Geometry check sheet. Reference: the model listing, model coordinates, mm. A direction names the side the tool comes from. Give positions to 0.01 mm unless a question says otherwise; leave off trailing zeros. Loops run counter-clockwise (first coordinate to the right, second up) from the corner with the lowest first, then second, coordinate; pieces in that order, holes last. Notation, with made-up numbers: (29.25, 69.5) -> (65.25, 69.5) arc R27 cw to (65.25, 90.5) -> close; hole circle Ø4 at (-24, 15.25). An arc over 180 degrees is marked (long way). One line per item, written item: value. Start each with the question number.
(1) Draft check along Z on faces 4 (the face through (0, 5, -33)), 5 (the face through (-4, 11.5, -18)), 6 (the face through (0, 7, -2)). Enter one of: pulls with the +Z half, pulls with the -Z half, needs draft (parallel to the pull), parting line crosses it, or undercut.
(2) Sectioned sample at D-D, the plane x = 0.25. Record the cut outline in (y, z), then the cut area to 3 significant figures.
(3) Gauge pin test, flat ends, axial feed: pin 1 Ø4.5 at (x, z) = (1, 0) entering from +Y; pin 2 Ø1.2 at (y, z) = (13, 0.5) entering from -X. Record the tip position at first contact, or that the pin passes through.
(4) Tool access check on faces 1 (the face through (0, 7, 2)), 2 (the face through (3.5, 13, 0)), 3 (the face through (-10.5, 2, 0)). Record the directions out of +Z, -Z, +X, -X, +Y, -Y that give a thin tool (end or side, any length) a straight path to the whole face; none if there is none.
(5) Sectioned sample at A-A, the plane y = 7.5. Record the cut outline in (x, z), then the cut area to 3 significant figures.
(6) Scan lines: line 1 along Z through (x, y) = (-1, 9); line 2 along X through (y, z) = (12.75, 9.5); line 3 along Y through (x, z) = (0, -21). Record each from-to range of solid material in increasing order. Write a range as from..to.
(7) Sectioned sample at C-C, the plane z = -0.5. Record the cut outline in (x, y), then the cut area to 3 significant figures.
(8) Sectioned sample at B-B, the plane x = 5.75. Record the cut outline in (y, z), then the cut area to 3 significant figures.
from build123d import *

# Parameters (mm, degrees)
SK_P01_CARRIER_W             = 21
SK_P01_CARRIER_H             = 66
P01_CARRIER_DEPTH            = 3
P02_WAGO221415GNDSTAR_START  = 3
SK_P02_WAGO221415GNDSTAR_W   = 21
SK_P02_WAGO221415GNDSTAR_H   = 31
P02_WAGO221415GNDSTAR_DEPTH  = 8.5
P03_WAGO221415PACKNODE_START = 3
SK_P03_WAGO221415PACKNODE_W  = 21
SK_P03_WAGO221415PACKNODE_H  = 31
P03_WAGO221415PACKNODE_DEPTH = 8.5
P04_LEVERS_START             = 11.5
SK_P04_LEVERS_W              = 7
SK_P04_LEVERS_H              = 66
P04_LEVERS_DEPTH             = 2.5


with BuildPart() as part:
    # SK_P01_Carrier → P01_Carrier (new body)
    with BuildSketch(Plane(origin=(0, 0, 0), x_dir=(1, 0, 0), z_dir=(0, 1, 0))):
        Rectangle(SK_P01_CARRIER_W, SK_P01_CARRIER_H)
    extrude(amount=P01_CARRIER_DEPTH)

    # SK_P02_WAGO221415GNDstar → P02_WAGO221415GNDstar (add)
    with BuildSketch(Plane(origin=(0, 0, 0), x_dir=(1, 0, 0), z_dir=(0, 1, 0)).offset(P02_WAGO221415GNDSTAR_START)):
        with Locations((0, 17.5)):
            Rectangle(SK_P02_WAGO221415GNDSTAR_W, SK_P02_WAGO221415GNDSTAR_H)
    extrude(amount=P02_WAGO221415GNDSTAR_DEPTH)

    # SK_P03_WAGO221415packnode → P03_WAGO221415packnode (add)
    with BuildSketch(Plane(origin=(0, 0, 0), x_dir=(1, 0, 0), z_dir=(0, 1, 0)).offset(P03_WAGO221415PACKNODE_START)):
        with Locations((0, -17.5)):
            Rectangle(SK_P03_WAGO221415PACKNODE_W, SK_P03_WAGO221415PACKNODE_H)
    extrude(amount=P03_WAGO221415PACKNODE_DEPTH)

    # SK_P04_Levers → P04_Levers (add)
    with BuildSketch(Plane(origin=(0, 0, 0), x_dir=(1, 0, 0), z_dir=(0, 1, 0)).offset(P04_LEVERS_START)):
        with Locations((7, 0)):
            Rectangle(SK_P04_LEVERS_W, SK_P04_LEVERS_H)
    extrude(amount=P04_LEVERS_DEPTH)


solid = part.part
Calculated:
1. face 4: pulls with the -Z half
1. face 5: needs draft
1. face 6: undercut
2. outline: (0, -33) -> (11.5, -33) -> (11.5, -2) -> (3, -2) -> (3, 2) -> (11.5, 2) -> (11.5, 33) -> (0, 33) -> close
2. area: 725 mm2
3. pin 1: stops at y = 11.5
3. pin 2: stops at x = 3.5
4. face 1: +X, -X
4. face 2: +Z, -Z, -X, +Y
4. face 3: +Z, -Z, -X, +Y, -Y
5. outline: (-10.5, -33) -> (10.5, -33) -> (10.5, -2) -> (-10.5, -2) -> close; (-10.5, 2) -> (10.5, 2) -> (10.5, 33) -> (-10.5, 33) -> close
5. area: 1,300 mm2
6. line 1: z = -33..-2, 2..33
6. line 2: x = 3.5..10.5
6. line 3: y = 0..11.5
7. outline: (-10.5, 0) -> (10.5, 0) -> (10.5, 3) -> (-10.5, 3) -> close; (3.5, 11.5) -> (10.5, 11.5) -> (10.5, 14) -> (3.5, 14) -> close
7. area: 80.5 mm2
8. outline: (0, -33) -> (14, -33) -> (14, 33) -> (0, 33) -> close; hole (3, -2) -> (11.5, -2) -> (11.5, 2) -> (3, 2) -> close
8. area: 890 mm2
